Geometry: final body of the model. Coordinates: model frame, mm. Round coordinates to 2 decimals unless told otherwise and drop trailing zeros. Order: outer loops, then holes, each group sorted by start corner. A loop starts at its lowest first (then second) coordinate and runs counter-clockwise, first axis right, second up. Notation, with made-up numbers: M -20.75,-33.75 L 38.25,-33.75 A31 cw 38.25,2.25 Z; hole C 18,-27.5 d7. An arc over 180 degrees is marked long. Return JSON: item names as keys, results as strings. Group by question number.
Q1. Cut plane D-D on x = -5.5. Output: boundary loops of the cut face in (y, z).
Q2. Cut plane B-B on y = 2.05. Output: boundary loops of the cut face in (x, z).
Q3. Contact query for flat-ended pins moving along their axis: pin 1 (3 mm diameter, centred on x = 50.78, z = -78.34, fed in from +Y); pin 2 (2 mm diameter, centred on y = 4, z = -37, fed in from +X); pin 3 (3 mm diameter, centred on y = 3.5, z = -89, fed in from +X). Output: stop coordinate, or through.
Q4. Cut plane C-C on z = -220. Output: boundary loops of the cut face in (x, y), and give its area (3 significant figures).
Q5. Mould query, pull axis Z, two halves, no side actions, for faces 1 (the face through (-7.93, 2.46, -41.24)), 2 (the face through (21.96, 2.46, -339.21)), 3 (the face through (24, 0, -177)). Classes: released by +Z, released by -Z, zero draft, split by the parting line, or undercut.
Q6. Ray query, probe 1 along Z at (x, y) = (21, 2.8); probe 2 along Z at (x, y) = (43, 2.5); probe 3 along X at (y, z) = (2.35, -166.5). Return the intervals inside material, ascending.
Q7. Cut plane A-A on x = 25. Output: boundary loops of the cut face in (y, z), and give its area (3 significant figures).
```python
from build123d import *

# Parameters (mm, degrees)
SKETCH1_R           = 2.5
SKETCH1_R_2         = 5
BOSS_EXTRUDE1_DEPTH = 5


with BuildPart() as part:
    # Sketch1 → Boss-Extrude1 (new body)
    with BuildSketch(Plane(origin=(0, 0, 0), x_dir=(1, 0, 0), z_dir=(0, 1, 0))):
        with BuildLine():
            Line((4.130127217, 0), (45.869872783, 0))
            ThreePointArc((45.869872783, 0), (49.054139071, 1.145074812), (50.779916111, 4.055820718))
            Line((50.779916111, 4.055820718), (64.883723024, 77.400263156))
            ThreePointArc((64.883723024, 77.400263156), (64.962312899, 78.007487301), (64.966093723, 78.619764391))
            Line((64.966093723, 78.619764391), (50.260556832, 345.275321952))
            ThreePointArc((50.260556832, 345.275321952), (48.704957481, 348.63157058), (45.268142804, 350))
            Line((45.268142804, 350), (4.731857196, 350))
            ThreePointArc((4.731857196, 350), (1.295042519, 348.63157058), (-0.260556832, 345.275321952))
            Line((-0.260556832, 345.275321952), (-14.966093723, 78.619764391))
            ThreePointArc((-14.966093723, 78.619764391), (-14.962312899, 78.007487301), (-14.883723024, 77.400263156))
            Line((-14.883723024, 77.400263156), (-0.779916111, 4.055820718))
            ThreePointArc((-0.779916111, 4.055820718), (0.945860929, 1.145074812), (4.130127217, 0))
        make_face()
        with Locations(Location((50.779916111, 78.344442439, 0), (0, 0, 270))):
            Circle(SKETCH1_R, mode=Mode.SUBTRACT)
        with Locations(Location((0, 78.344442439, 0), (0, 0, 270))):
            Circle(SKETCH1_R, mode=Mode.SUBTRACT)
        with Locations(Location((25, 11.876781334, 0), (0, 0, 270))):
            Circle(SKETCH1_R_2, mode=Mode.SUBTRACT)
        with Locations(Location((45.268142804, 213.58952196, 0), (0, 0, 270))):
            Circle(SKETCH1_R, mode=Mode.SUBTRACT)
        with Locations(Location((4.731857196, 213.58952196, 0), (0, 0, 270))):
            Circle(SKETCH1_R, mode=Mode.SUBTRACT)
        with Locations(Location((25, 335.239262598, 0), (0, 0, 270))):
            Circle(SKETCH1_R_2, mode=Mode.SUBTRACT)
    extrude(amount=BOSS_EXTRUDE1_DEPTH)


solid = part.part
```
Result sheet:
{
 "1": {"outline": "M 0,-250.27 L 5,-250.27 L 5,-28.6 L 0,-28.6 Z"},
 "2": {"outline": "M -14.97,-78.62 L -0.26,-345.28 A5 ccw 4.73,-350 L 45.27,-350 A5 ccw 50.26,-345.28 L 64.97,-78.62 A5 ccw 64.88,-77.4 L 50.78,-4.06 A5 ccw 45.87,0 L 4.13,0 A5 ccw -0.78,-4.06 L -14.88,-77.4 A5 ccw Z; hole C 0,-78.34 d5; hole C 4.73,-213.59 d5; hole C 25,-335.24 d10; hole C 25,-11.88 d10; hole C 45.27,-213.59 d5; hole C 50.78,-78.34 d5"},
 "3": {"pin 1": "passes through", "pin 2": "stops at x = 57.31", "pin 3": "stops at x = 64.48"},
 "4": {"outline": "M -7.17,0 L 57.17,0 L 57.17,5 L -7.17,5 Z", "area": "322 mm²"},
 "5": {"face 1": "released by +Z", "face 2": "undercut", "face 3": "zero draft"},
 "6": {"probe 1": "z = -350 to -338.24, -332.24 to -14.88, -8.88 to 0", "probe 2": "z = -350 to -214.64, -212.54 to 0", "probe 3": "x = -10.12 to 60.12"},
 "7": {"outline": "M 0,-350 L 5,-350 L 5,-340.24 L 0,-340.24 Z; M 0,-330.24 L 5,-330.24 L 5,-16.88 L 0,-16.88 Z; M 0,-6.88 L 5,-6.88 L 5,0 L 0,0 Z", "area": "1,650 mm²"}
}
